Autodesk Inventor part; units mm, degrees
ref_plane "Work Plane1" through (22, 0, 0) normal (1, 0, 0) x (0, 1, 0)
ref_plane "YZ Plane" through (0, 0, 0) normal (1, 0, 0) x (0, 1, 0)
ref_plane "XZ Plane" through (0, 0, 0) normal (0, 1, 0) x (-1, 0, 0)
sketch "Sketch1" plane through (0, 0, 0) normal (0, 0, 1) x (1, 0, 0)
  line L0 (0, 0) -> (44, 0)
  line L1 (0, 0) -> (0, 8.5) construction
  line L2 (22, 4.5) -> (22, 8.5)
  line L3 (44, 4.5) -> (44, 0) construction
  line L4 (0, 8.5) -> (0, 10.2225)
  line L5 (44, 4.5) -> (44, 6.3907)
  line L6 (36, 6.6407) -> (36, 4.5) construction
  line L7 (18, 13) -> (26, 13)
  line L8 (22, 8.5) -> (22, 13) construction
  line L9 (22, 8.5) -> (0, 8.5)
  line L10 (22, 4.5) -> (44, 4.5)
  line L11 (0, 10.2225) -> (11, 10.5663)
  line L12 (11, 10.5663) -> (11, 8.5) construction
  line L13 (11, 10.5663) -> (18, 10.5663)
  line L14 (18, 10.5663) -> (18, 13)
  line L15 (44, 6.3907) -> (36, 6.6407)
  line L16 (26, 6.6407) -> (26, 13) construction
  line L17 (22, 4.5) -> (22, 0) construction
  line L18 (26, 13) -> (27.704, 6.6407)
  line L19 (36, 6.6407) -> (27.704, 6.6407)
  line L20 (26, 6.6407) -> (27.704, 6.6407) construction
  line L21 (37.99, 6.5785) -> (37.99, 0) construction
  line L22 (8.16, 10.4775) -> (8.16, 0) construction
  line L23 (11, 8.5) -> (11, 0) construction
  line L24 (36, 4.5) -> (36, 0) construction
  dimension "d0" = 44
  dimension "d3" = 26
  dimension "d4" = 9
  dimension "d5" = 1.79
  dimension "d6" = 17
  dimension "d7" = 1.79
  dimension "d8" = 11
  dimension "d9" = 8
  dimension "d10" = 8
  dimension "d14" = 15
  dimension "d16" = 8.16
  dimension "d17" = 6.01
  dimension "d18" = 13.157
  dimension "d23" = 20.955
revolve "Revolve1" add sketch "Sketch1" angle 360 about axis through (0, 0, 0) along (1, 0, 0)
ref_plane "Work Plane1" through (22, 0, 0) normal (1, 0, 0) x (0, 1, 0)
sketch "Sketch2" plane through (22, 0, 0) normal (1, 0, 0) x (0, 1, 0)
  line L0 (0, -15.0111) -> (-13, -7.5056)
  line L1 (-13, -7.5056) -> (-13, 7.5056)
  line L2 (-13, 7.5056) -> (0, 15.0111)
  line L3 (0, 15.0111) -> (13, 7.5056)
  line L4 (13, 7.5056) -> (13, -7.5056)
  line L5 (13, -7.5056) -> (0, -15.0111)
  circle A0 centre (0, 0) radius 13
  circle A1 centre (0, 0) radius 13
extrude "Extrude1" add sketch "Sketch2" along normal mid plane 8 contours L0 A0 L5 | L0 L1 A0 | A0 L4 L5 | L1 L2 A0 | A0 L3 L4 | L2 L3 A0
thread "Thread1"
thread "Thread2"
equation "\"d0\" = L"
equation "\"d3\" = S"
equation "\"d4\" = A32 - 2 * t2"
equation "\"d6\" = A31 - 2 * t1"
equation "\"d8\" = L1"
equation "\"d9\" = M"
equation "\"d10\" = L2"
equation "\"d16\" = A1"
equation "\"d17\" = A2"
equation "\"d18\" = OD2"
equation "\"d23\" = OD1"
equation "\"d12\" = M"
equation "\"OD1\" = 20.955"
equation "\"OD2\" = 13.157"
equation "\"L\" = 44"
equation "\"M\" = 8"
equation "\"S\" = 26"
equation "\"L1\" = 11"
equation "\"L2\" = 8"
equation "\"d11\" = 0.5 * L"
equation "\"A1\" = 8.16"
equation "\"A2\" = 6.01"
equation "\"A31\" = 22"
equation "\"A32\" = 14"
equation "\"t1\" = 2.5"
equation "\"t2\" = 2.5"
equation "\"Size_Designation\" = 1.2345"
properties part number "JIS B 2301 Reducing Hexagon Nipple - Class II 1/2 x 1/4" material "Iron, Cast"
Geometry: final body of the model. Coordinates: model frame, mm. A direction names the side the tool comes from. Round coordinates to 2 decimals unless told otherwise and drop trailing zeros. Loops run counter-clockwise (first coordinate to the right, second up) from the corner with the lowest first, then second, coordinate; pieces in that order, holes last. Notation, with made-up numbers: M -20,6.25 L -4,6.25 A19 ccw -4,14.25 Z; hole C -31.75,68.25 d7. An arc over 180 degrees is marked long. Put each result on its own line as item: value. Start each with the question number.
(1) Draft query along Y for faces 4 (the face through (22, 4, -4)), 5 (the face through (21.9, 6.6, -11.2)), 6 (the face through (33.15, -0.59, 4.46)), 7 (the face through (14.549, -2.291, -10.315)). Return one class per face: +Y half, -Y half, draft (parallel to the pull), parting line (faces both ways), or undercut.
(2) Section query A-A (x = 24.5). Return loops of the section in (y, z).
(3) Material intervals for line 1 along Z through (x, y) = (34, 0); line 2 along Z through (x, y) = (13.25, 0); line 3 along X through (y, z) = (11.5, 6), sorted ascending. Write a range as [from, to].
(4) Section query C-C (x = 3). Return loops of the section in (y, z).
(5) Set-up query: faces 1 (the face through (26, 12, -7)), 2 (the face through (31.794, 3.064, 5.891)), 3 (the face through (18, -4, -10)). Return all of +Z, -Z, +X, -X, +Y, -Y with unobstructed straight access to the full face (end or side cutting, diameter ignored); none if empty.
(6) Section query B-B (x = 39.5). Return loops of the section in (y, z), then the cut area to 3 significant figures.
(7) Contact query for flat-ended pins moving along their axis: pin 1 Ø3 at (y, z) = (-9.5, -8) entering from +X; pin 2 Ø5 at (x, y) = (8, 7) entering from +Z; pin 3 Ø2 at (x, z) = (13.5, 4.5) entering from +Y; pin 4 Ø6 at (x, y) = (37, 10) entering from +Z. Output: stop coordinate, or through.
Findings below:
1. face 4: undercut
1. face 5: +Y half
1. face 6: undercut
1. face 7: parting line
2. outline: M -13,-7.51 L 0,-15.01 L 13,-7.51 L 13,7.51 L 0,15.01 L -13,7.51 Z; hole C 0,0 d9
3. line 1: z = [-6.64, -4.5], [4.5, 6.64]
3. line 2: z = [-10.57, -8.5], [8.5, 10.57]
3. line 3: x = [18, 26.01]
4. outline: C 0,0 d20.63; hole C 0,0 d17
5. face 1: -Z, +X, +Y
5. face 2: +X
5. face 3: -X
6. outline: C 0,0 d13.06; hole C 0,0 d9
6. area: 70.4 mm2
7. pin 1: stops at x = 26.56
7. pin 2: stops at z = 9.46
7. pin 3: stops at y = 9.97
7. pin 4: passes through
